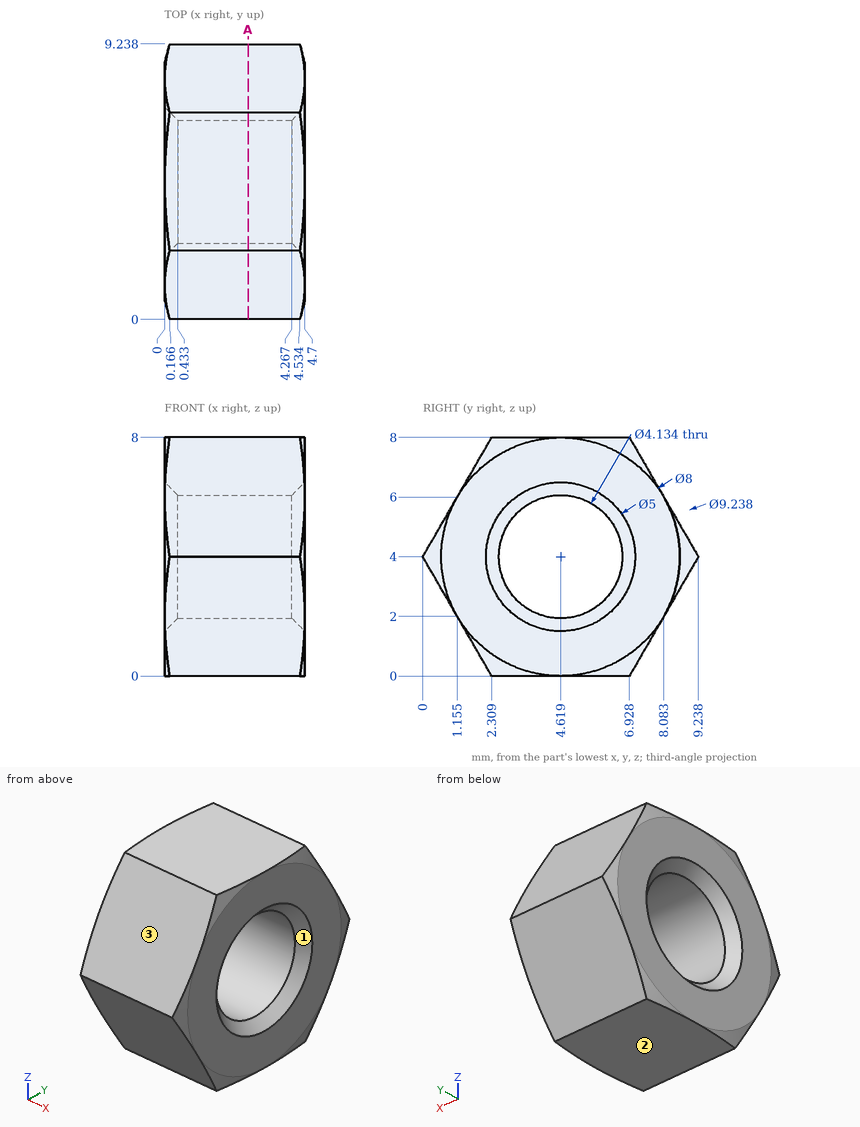
The drawing under review shows one solid part. Ordinate dimensions are in mm from its lowest x, y, z. Coordinates: 2 decimals unless noted, no trailing zeros. Write each loop counter-clockwise with the first axis right and the second up, starting at its lowest first coordinate (ties: lowest second). Pieces come first, ordered by that corner, then holes. Notation, with made-up numbers: (75.25, 61) - (123.25, 61) arc R15 ccw to (123.25, 85) - close; hole circle Ø7 at (18.5, 35). An arc over 180 degrees is marked (long way). Put each result on its own line as item: value.
1. Wall thickness on probe 1 along Z at (x, y) = (0.25, 5.5); probe 2 along Z at (x, y) = (0.4, 2.75) (1 decimal); probe 3 along Y at (x, z) = (1.1, 4.75) (1 decimal): over which ranges is each line inside the solid? List them lowest first.
Values found:
probe 1: 0 to 1.93, 6.07 to 8
probe 2: 0 to 3, 5 to 8
probe 3: 0.4 to 2.7, 6.5 to 8.8
2. Mouldability with a two-part tool opening along Y and no side actions: class the marked faces 1, 2 and 3 as released by +Y, released by -Y, zero draft, split by the parting line, or undercut.
Values found:
face 1: undercut
face 2: zero draft
face 3: released by -Y
3. Add section A-A, the plane x = 2.8. Give the boundary of the cut face in (y, z) (1 decimal), then the cut area to 3 significant figures.
Values found:
outline: (0, 4) - (2.3, 0) - (6.9, 0) - (9.2, 4) - (6.9, 8) - (2.3, 8) - close; hole circle Ø4.1 at (4.6, 4)
area: 42.0 mm²
4. For pin 1 (1.5 mm diameter, centred on x = 3, z = 6, fed in from +Y) (1 decimal); pin 2 (1 mm diameter, centred on y = 2, z = 1, fed in from -X), all flat-tipped, find the tip position at first contact; note any pin that passes through.
Values found:
pin 1: y = 8.5
pin 2: x = 0
